from build123d import *

# Parameters (mm, degrees)
PAD001_DEPTH = 2
SKETCH002_R  = 1
POCKET_DEPTH = 5
CHAMFER_SIZE = 1


with BuildPart() as part:
    # Sketch001 → Pad001 (new body, symmetric)
    with BuildSketch(Plane.YZ):
        with BuildLine():
            Line((-0.2, 0), (-0.2, 7.928203))
            ThreePointArc((-0.2, 7.928203), (-0.336297, 8.963479), (-0.735898, 9.928203))
            Line((-0.735898, 9.928203), (-1.2, 10.732051))
            ThreePointArc((-1.12969, 12.342415), (-1.399534, 11.54748), (-1.2, 10.732051))
            Line((-1.12969, 12.342415), (0.965775, 15.335049))
            ThreePointArc((0.965775, 15.335049), (1.181471, 16.006654), (0.980132, 16.682702))
            Line((0.980132, 16.682702), (-0.255119, 18.529347))
            Line((-0.255119, 18.529347), (0, 18.7))
            Line((0, 18.7), (1.235251, 16.853356))
            ThreePointArc((1.2172, 15.158999), (1.488387, 16.003385), (1.235251, 16.853356))
            Line((1.2172, 15.158999), (-0.728007, 12.380955))
            ThreePointArc((-0.728007, 12.380955), (-1.00431, 11.566995), (-0.8, 10.732051))
            Line((-0.8, 10.732051), (-0.335898, 9.928203))
            ThreePointArc((0.2, 7.928203), (0.063703, 8.963479), (-0.335898, 9.928203))
            Line((0.2, 7.928203), (0.2, 0))
            Line((-0.2, 0), (0.2, 0))
        make_face()
    extrude(amount=PAD001_DEPTH, both=True)

    # Sketch002 (on Face1 of Pad001) → Pocket (cut)
    with BuildSketch(Plane.ZX.offset(0.2)):
        with Locations((2, 0)):
            Circle(SKETCH002_R)
    extrude(amount=-POCKET_DEPTH, mode=Mode.SUBTRACT)

    # Chamfer
    chamfer_edges = [part.edges().sort_by_distance(p)[0] for p in [
        (2, 0, 0),
        (-2, 0, 0),
    ]]
    chamfer(chamfer_edges, length=CHAMFER_SIZE)


solid = part.part
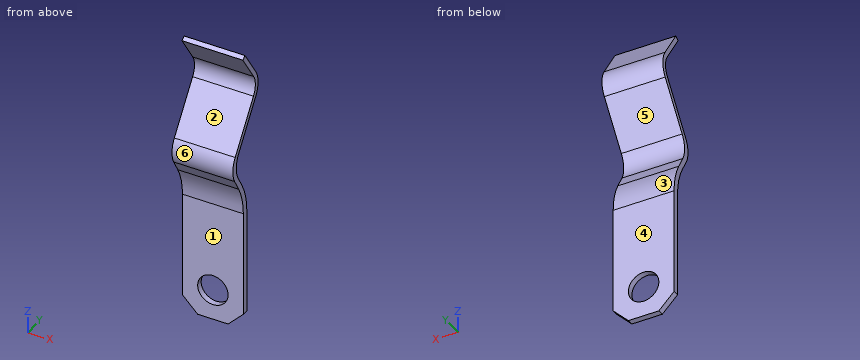
Could you check a few things on this model? Use its own coordinates, in mm. Face numbers are marked on the shaded views. A direction names the side the tool comes from. Coordinates: 2 decimals unless noted, no trailing zeros. Loops run counter-clockwise (first coordinate to the right, second up) from the corner with the lowest first, then second, coordinate; pieces in that order, holes last.
1. Imagine slicing it at D-D (x = 1.7). Please give me the cut outline in (y, z).
2. Imagine slicing it at C-C (y = 0.7). Please give me the cut outline in (x, z), and give its area (3 significant figures).
3. For P1, Ø1.2, axis at x = 0, z = 2.5, coming from the -Y side; P2, Ø1.5, axis at x = -1, z = 9, coming from the -Y side, each with a flat end and sliding along its axis, tell me the tip position at first contact or that it passes through.
4. Imagine slicing it at B-B (x = 0.6). Please give me the cut outline in (y, z), and give its area (3 significant figures).
5. For the marked faces 1, 2 and 3, which set-ups out of +Z, -Z, +X, -X, +Y, -Y let a thin tool reach every point of the face, with its end or its side?
6. I need wall thicknesses on L1, parallel to X at y = 0.05, z = 2; L2, parallel to Y at x = 0.5, z = 5.75; L3, parallel to Y at x = 0.85, z = 13. Which ranges of each line are inside material? Lowest first, please.
7. Imagine slicing it at A-A (z = 2). Please give me the cut outline in (x, y).
8. We'd pull the mould along Z, two halves only. Please class the marked faces 4, 5 and 6: released by +Z, released by -Z, zero draft, split by the parting line, or undercut.
Computed values:
1. outline: (-1.2, 10.73) - (-0.74, 9.93) arc R4 cw to (-0.2, 7.93) - (-0.2, 0.7) - (0.2, 0.7) - (0.2, 7.93) arc R4 ccw to (-0.34, 9.93) - (-0.8, 10.73) arc R1.54 cw to (-0.73, 12.38) - (1.22, 15.16) arc R1.5 ccw to (1.24, 16.85) - (0, 18.7) - (-0.26, 18.53) - (0.98, 16.68) arc R1.19 cw to (0.97, 15.34) - (-1.13, 12.34) arc R1.5 ccw to start
2. outline: (-2, 14.42) - (2, 14.42) - (2, 14.96) - (-2, 14.96) - close; (-2, 17.1) - (2, 17.1) - (2, 17.65) - (-2, 17.65) - close
2. area: 4.35 mm2
3. P1: stops at y = -0.2
3. P2: stops at y = -0.64
4. outline: (-1.2, 10.73) - (-0.74, 9.93) arc R4 cw to (-0.2, 7.93) - (-0.2, 2.8) - (0.2, 2.8) - (0.2, 7.93) arc R4 ccw to (-0.34, 9.93) - (-0.8, 10.73) arc R1.54 cw to (-0.73, 12.38) - (1.22, 15.16) arc R1.5 ccw to (1.24, 16.85) - (0, 18.7) - (-0.26, 18.53) - (0.98, 16.68) arc R1.19 cw to (0.97, 15.34) - (-1.13, 12.34) arc R1.5 ccw to start; (-0.2, 0) - (0.2, 0) - (0.2, 1.2) - (-0.2, 1.2) - close
4. area: 6.55 mm2
5. face 1: -Z, +X, -X, -Y
5. face 2: +X, -X, -Y
5. face 3: +X, -X, +Y
6. L1: x = -2 to -1, 1 to 2
6. L2: y = -0.2 to 0.2
6. L3: y = -0.67 to -0.29
7. outline: (-2, -0.2) - (-1, -0.2) - (-1, 0.2) - (-2, 0.2) - close; (1, -0.2) - (2, -0.2) - (2, 0.2) - (1, 0.2) - close
8. face 4: zero draft
8. face 5: undercut
8. face 6: split by the parting line
